Geometry check sheet. Reference: the model listing, model coordinates, mm. Face numbers are marked on the shaded views. Coordinates: 2 decimals unless noted, no trailing zeros. Write each loop counter-clockwise with the first axis right and the second up, starting at its lowest first coordinate (ties: lowest second). Pieces come first, ordered by that corner, then holes.
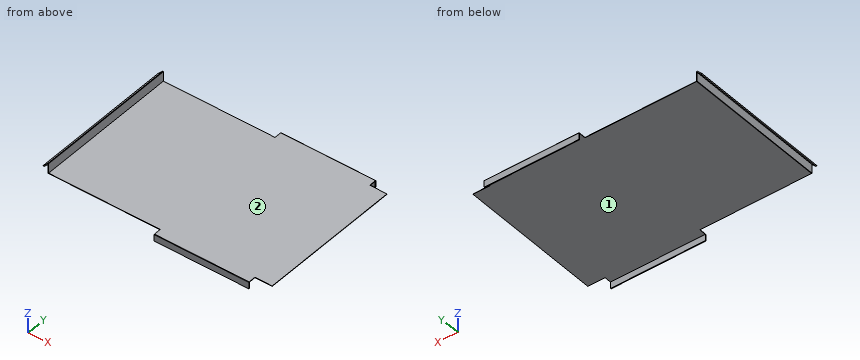
from build123d import *

# Parameters (mm, degrees)
F1_DEPTH  = 1.25
F2_W      = 275
F2_H      = 2
F3_DEPTH  = 20
F4_W      = 1.25
F4_H      = 420
F5_DEPTH  = 30
F6_W      = 420
F6_H      = 15
F7_DEPTH  = 15
F8_SIZE   = 14.99999
F10_R     = 1
F11_R     = 1
F12_DEPTH = 442.001


# Not quite as in the source:
# - a fillet or chamfer is up to 0.001 mm smaller than in the source, because OpenCascade refuses the exact size


with BuildPart() as f1:
    # F0 (on Top) → F1 (new body)
    with BuildSketch(Plane.XY):
        Polygon((0, -232), (275, -232), (275, -210), (325, -210), (325, 210), (275, 210), (275, 232), (0, 232), (0, 210), (-325, 210), (-325, -210), (0, -210), align=None)
    extrude(amount=F1_DEPTH)

    # F2 (on face) → F3 (join)
    with BuildSketch(Plane.XY.offset(1.25)):
        with Locations((137.5, 231)):
            Rectangle(F2_W, F2_H)
        with Locations((137.5, -231)):
            Rectangle(F2_W, F2_H)
    extrude(amount=-F3_DEPTH)

    # F4 (on face) → F5 (join)
    with BuildSketch(Plane(origin=(0, 0, 0), x_dir=(1, 0, 0), z_dir=(0, 0, -1))):
        with Locations((-324.375, 0)):
            Rectangle(F4_W, F4_H)
    extrude(amount=-F5_DEPTH)

    # F6 (on face) → F7 (join)
    with BuildSketch(Plane(origin=(-325, 0, 0), x_dir=(0, -1, 0), z_dir=(-1, 0, 0))):
        with Locations((0, 22.5)):
            Rectangle(F6_W, F6_H)
    extrude(amount=F7_DEPTH)

    # F8 (size 15 in the source; OpenCascade refuses exactly that, so slightly less here)
    f8_edges = [f1.edges().sort_by_distance(p)[0] for p in [
        (-340, 0, 30),
    ]]
    chamfer(f8_edges, length=F8_SIZE)

    # F10
    f10_edges = [f1.edges().sort_by_distance(p)[0] for p in [
        (-323.75, 0, 30),
    ]]
    fillet(f10_edges, radius=F10_R)

    # F11
    f11_edges = [f1.edges().sort_by_distance(p)[0] for p in [
        (-325, 0, 0),
        (137.5, 232, 1.25),
        (137.5, -232, 1.25),
    ]]
    fillet(f11_edges, radius=F11_R)

    # F9 (on face) → F12 (cut, through all)
    with BuildSketch(Plane(origin=(0, 210, 0), x_dir=(-1, 0, 0), z_dir=(0, 1, 0))):
        Polygon((336.4644660941, 15), (325, 26.4644660941), (325, 15), align=None)
    extrude(amount=-F12_DEPTH, mode=Mode.SUBTRACT)


solid = f1.part
1. Thickness scan on line 1 along Y through (x, z) = (216, -14.5); line 2 along Z through (x, y) = (-116, 111); line 3 along X through (y, z) = (73, 3). Record the ranges inside material, lowest first.
Computed values:
line 1: y = -232 to -230, 230 to 232
line 2: z = 0 to 1.25
line 3: x = -325 to -323.75
2. Gauge pin test, flat ends, axial feed: pin 1 Ø1.1 at (x, y) = (-338.5, -103.5) entering from -Z; pin 2 Ø10 at (y, z) = (-66.5, 11.5) entering from +X; pin 3 Ø22 at (y, z) = (-222, -11.5) entering from +X. Record the tip position at first contact, or that the pin passes through.
Computed values:
pin 1: stops at z = 15
pin 2: stops at x = -323.75
pin 3: stops at x = 275
3. Draft check along Y on the marked faces 1 and 2. Enter one of: released by +Y, released by -Y, zero draft, split by the parting line, or undercut.
Computed values:
face 1: undercut
face 2: zero draft
4. Sectioned sample at C-C, the plane x = -164.5. Record the boundary of the cut face in (y, z), and give its area (3 significant figures).
Computed values:
outline: (-210, 0) - (210, 0) - (210, 1.25) - (-210, 1.25) - close
area: 525 mm2
5. Sectioned sample at A-A, the plane z = -9.5. Record the boundary of the cut face in (x, y), and give its area (3 significant figures).
Computed values:
outline: (0, -232) - (275, -232) - (275, -230) - (0, -230) - close; (0, 230) - (275, 230) - (275, 232) - (0, 232) - close
area: 1,100 mm2
